Here's how the part is built. I have some questions about the finished solid (model axes, mm). A direction names the side the tool comes from. Round coordinates to 2 decimals unless told otherwise and drop trailing zeros. Write each loop counter-clockwise with the first axis right and the second up, starting at its lowest first coordinate (ties: lowest second). Pieces come first, ordered by that corner, then holes. Notation, with made-up numbers: (68, 78) -> (105, 78) arc R16 ccw to (105, 102) -> close; hole circle Ø3 at (-16.5, -23). An arc over 180 degrees is marked (long way). Answer as CSV lines item,"result".
from build123d import *

# Parameters (mm, degrees)
SKETCH_1_R          = 13.5
SKETCH_1_R_2        = 1.6
EXTRUDE_1_DEPTH     = 3
CUT_EXTRUDE_START   = -10
CUT_EXTRUDE_1_DEPTH = 10
SKETCH_3_W          = 59.8
SKETCH_3_H          = 5
EXTRUDE_1_2_DEPTH   = 3
FILLET_1_R          = 2
SKETCH_4_R          = 1.6
CUT_EXTRUDE_2_DEPTH = 10


with BuildPart() as part:
    # 草图1 → Extrude 1 (new body)
    with BuildSketch(Plane(origin=(0, 0, 0), x_dir=(1, 0, 0), z_dir=(0, 1, 0))):
        with BuildLine():
            Line((-49, -44), (49, -44))
            ThreePointArc((49, -44), (70, -65), (49, -86))
            Line((49, -86), (-49, -86))
            ThreePointArc((-49, -86), (-70, -65), (-49, -44))
        make_face()
        with Locations(Location((-49, -65, 0), (0, 0, 270))):
            Circle(SKETCH_1_R, mode=Mode.SUBTRACT)
        with Locations(Location((49, -65, 0), (0, 0, 270))):
            Circle(SKETCH_1_R, mode=Mode.SUBTRACT)
        with Locations(Location((-49, -82.5, 0), (0, 0, 270))):
            Circle(SKETCH_1_R_2, mode=Mode.SUBTRACT)
        with Locations(Location((-57.75, -80.155444566, 0), (0, 0, 270))):
            Circle(SKETCH_1_R_2, mode=Mode.SUBTRACT)
        with Locations(Location((-64.155444566, -73.75, 0), (0, 0, 270))):
            Circle(SKETCH_1_R_2, mode=Mode.SUBTRACT)
        with Locations(Location((-66.5, -65, 0), (0, 0, 270))):
            Circle(SKETCH_1_R_2, mode=Mode.SUBTRACT)
        with Locations(Location((-64.155444566, -56.25, 0), (0, 0, 270))):
            Circle(SKETCH_1_R_2, mode=Mode.SUBTRACT)
        with Locations(Location((-57.75, -49.844555434, 0), (0, 0, 270))):
            Circle(SKETCH_1_R_2, mode=Mode.SUBTRACT)
        with Locations(Location((-49, -47.5, 0), (0, 0, 270))):
            Circle(SKETCH_1_R_2, mode=Mode.SUBTRACT)
        with Locations(Location((-40.25, -49.844555434, 0), (0, 0, 270))):
            Circle(SKETCH_1_R_2, mode=Mode.SUBTRACT)
        with Locations(Location((-33.844555434, -56.25, 0), (0, 0, 270))):
            Circle(SKETCH_1_R_2, mode=Mode.SUBTRACT)
        with Locations(Location((-31.5, -65, 0), (0, 0, 270))):
            Circle(SKETCH_1_R_2, mode=Mode.SUBTRACT)
        with Locations(Location((-33.844555434, -73.75, 0), (0, 0, 270))):
            Circle(SKETCH_1_R_2, mode=Mode.SUBTRACT)
        with Locations(Location((-40.25, -80.155444566, 0), (0, 0, 270))):
            Circle(SKETCH_1_R_2, mode=Mode.SUBTRACT)
        with Locations(Location((64.155444566, -56.25, 0), (0, 0, 270))):
            Circle(SKETCH_1_R_2, mode=Mode.SUBTRACT)
        with Locations(Location((66.5, -65, 0), (0, 0, 270))):
            Circle(SKETCH_1_R_2, mode=Mode.SUBTRACT)
        with Locations(Location((64.155444566, -73.75, 0), (0, 0, 270))):
            Circle(SKETCH_1_R_2, mode=Mode.SUBTRACT)
        with Locations(Location((57.75, -80.155444566, 0), (0, 0, 270))):
            Circle(SKETCH_1_R_2, mode=Mode.SUBTRACT)
        with Locations(Location((49, -82.5, 0), (0, 0, 270))):
            Circle(SKETCH_1_R_2, mode=Mode.SUBTRACT)
        with Locations(Location((40.25, -80.155444566, 0), (0, 0, 270))):
            Circle(SKETCH_1_R_2, mode=Mode.SUBTRACT)
        with Locations(Location((33.844555434, -73.75, 0), (0, 0, 270))):
            Circle(SKETCH_1_R_2, mode=Mode.SUBTRACT)
        with Locations(Location((31.5, -65, 0), (0, 0, 270))):
            Circle(SKETCH_1_R_2, mode=Mode.SUBTRACT)
        with Locations(Location((33.844555434, -56.25, 0), (0, 0, 270))):
            Circle(SKETCH_1_R_2, mode=Mode.SUBTRACT)
        with Locations(Location((40.25, -49.844555434, 0), (0, 0, 270))):
            Circle(SKETCH_1_R_2, mode=Mode.SUBTRACT)
        with Locations(Location((49, -47.5, 0), (0, 0, 270))):
            Circle(SKETCH_1_R_2, mode=Mode.SUBTRACT)
        with Locations(Location((57.75, -49.844555434, 0), (0, 0, 270))):
            Circle(SKETCH_1_R_2, mode=Mode.SUBTRACT)
        with Locations(Location((13, -52, 0), (0, 0, 270))):
            Circle(SKETCH_1_R_2, mode=Mode.SUBTRACT)
        with Locations(Location((-13, -52, 0), (0, 0, 270))):
            Circle(SKETCH_1_R_2, mode=Mode.SUBTRACT)
        with Locations(Location((13, -78, 0), (0, 0, 270))):
            Circle(SKETCH_1_R_2, mode=Mode.SUBTRACT)
        with Locations(Location((-13, -78, 0), (0, 0, 270))):
            Circle(SKETCH_1_R_2, mode=Mode.SUBTRACT)
    extrude(amount=EXTRUDE_1_DEPTH)

    # 草图2 → 切除-拉伸1 (cut)
    with BuildSketch(Plane(origin=(0, 3, 0), x_dir=(1, 0, 0), z_dir=(0, 1, 0)).offset(CUT_EXTRUDE_START)):
        with BuildLine():
            Line((-16.872983346, -51), (-33.347524158, -51))
            ThreePointArc((-33.347524158, -51), (-29.382380462, -57.506736115), (-28, -65))
            ThreePointArc((-28, -65), (-29.382380462, -72.493263885), (-33.347524158, -79))
            Line((-33.347524158, -79), (-16.872983346, -79))
            ThreePointArc((-16.872983346, -79), (-13.50401717, -74.031881215), (-9, -78))
            ThreePointArc((-9, -78), (-9.031881215, -78.50401717), (-9.127016654, -79))
            Line((-9.127016654, -79), (9.127016654, -79))
            ThreePointArc((9.127016654, -79), (12.49598283, -74.031881215), (17, -78))
            ThreePointArc((17, -78), (16.968118785, -78.50401717), (16.872983346, -79))
            Line((16.872983346, -79), (33.347524158, -79))
            ThreePointArc((33.347524158, -79), (28, -65), (33.347524158, -51))
            Line((33.347524158, -51), (16.872983346, -51))
            ThreePointArc((16.872983346, -51), (16.968118785, -51.49598283), (17, -52))
            ThreePointArc((17, -52), (12.49598283, -55.968118785), (9.127016654, -51))
            Line((9.127016654, -51), (-9.127016654, -51))
            ThreePointArc((-9.127016654, -51), (-9.031881215, -51.49598283), (-9, -52))
            ThreePointArc((-9, -52), (-13.50401717, -55.968118785), (-16.872983346, -51))
        make_face()
        with BuildLine():
            ThreePointArc((17, -78), (12.49598283, -74.031881215), (9.127016654, -79))
            Line((9.127016654, -79), (11.7510004, -79))
            ThreePointArc((11.7510004, -79), (12.470094046, -76.490298149), (14.6, -78))
            ThreePointArc((14.6, -78), (14.509701851, -78.529905954), (14.2489996, -79))
            Line((14.2489996, -79), (16.872983346, -79))
            ThreePointArc((16.872983346, -79), (16.968118785, -78.50401717), (17, -78))
        make_face()
        with BuildLine():
            Line((11.7510004, -79), (9.127016654, -79))
            ThreePointArc((9.127016654, -79), (13, -82), (16.872983346, -79))
            Line((16.872983346, -79), (14.2489996, -79))
            ThreePointArc((14.2489996, -79), (13, -79.6), (11.7510004, -79))
        make_face()
        with BuildLine():
            ThreePointArc((-9.127016654, -51), (-13, -48), (-16.872983346, -51))
            Line((-16.872983346, -51), (-14.2489996, -51))
            ThreePointArc((-14.2489996, -51), (-13, -50.4), (-11.7510004, -51))
            Line((-11.7510004, -51), (-9.127016654, -51))
        make_face()
        with BuildLine():
            Line((-14.2489996, -51), (-16.872983346, -51))
            ThreePointArc((-16.872983346, -51), (-13.50401717, -55.968118785), (-9, -52))
            ThreePointArc((-9, -52), (-9.031881215, -51.49598283), (-9.127016654, -51))
            Line((-9.127016654, -51), (-11.7510004, -51))
            ThreePointArc((-11.7510004, -51), (-11.490298149, -51.470094046), (-11.4, -52))
            ThreePointArc((-11.4, -52), (-13.529905954, -53.509701851), (-14.2489996, -51))
        make_face()
        with BuildLine():
            ThreePointArc((16.872983346, -51), (13, -48), (9.127016654, -51))
            Line((9.127016654, -51), (11.7510004, -51))
            ThreePointArc((11.7510004, -51), (13, -50.4), (14.2489996, -51))
            Line((14.2489996, -51), (16.872983346, -51))
        make_face()
        with BuildLine():
            Line((11.7510004, -51), (9.127016654, -51))
            ThreePointArc((9.127016654, -51), (12.49598283, -55.968118785), (17, -52))
            ThreePointArc((17, -52), (16.968118785, -51.49598283), (16.872983346, -51))
            Line((16.872983346, -51), (14.2489996, -51))
            ThreePointArc((14.2489996, -51), (14.509701851, -51.470094046), (14.6, -52))
            ThreePointArc((14.6, -52), (12.470094046, -53.509701851), (11.7510004, -51))
        make_face()
        with BuildLine():
            ThreePointArc((-9, -78), (-13.50401717, -74.031881215), (-16.872983346, -79))
            Line((-16.872983346, -79), (-14.2489996, -79))
            ThreePointArc((-14.2489996, -79), (-13.529905954, -76.490298149), (-11.4, -78))
            ThreePointArc((-11.4, -78), (-11.490298149, -78.529905954), (-11.7510004, -79))
            Line((-11.7510004, -79), (-9.127016654, -79))
            ThreePointArc((-9.127016654, -79), (-9.031881215, -78.50401717), (-9, -78))
        make_face()
        with BuildLine():
            Line((-14.2489996, -79), (-16.872983346, -79))
            ThreePointArc((-16.872983346, -79), (-13, -82), (-9.127016654, -79))
            Line((-9.127016654, -79), (-11.7510004, -79))
            ThreePointArc((-11.7510004, -79), (-13, -79.6), (-14.2489996, -79))
        make_face()
    extrude(amount=CUT_EXTRUDE_1_DEPTH, mode=Mode.SUBTRACT)

    # 草图3 → Extrude 1 2 (add)
    with BuildSketch(Plane(origin=(0, 3, 0), x_dir=(1, 0, 0), z_dir=(0, 1, 0))):
        with Locations((0, -65)):
            Rectangle(SKETCH_3_W, SKETCH_3_H)
    extrude(amount=-EXTRUDE_1_2_DEPTH)

    # 圆角1
    fillet_1_edges = [part.edges().sort_by_distance(p)[0] for p in [
        (-33.347524158, 1.5, 79),
        (-33.347524158, 1.5, 51),
        (-16.872983346, 1.5, 51),
        (-9.127016654, 1.5, 51),
        (9.127016654, 1.5, 51),
        (16.872983346, 1.5, 51),
        (33.347524158, 1.5, 51),
        (33.347524158, 1.5, 79),
        (16.872983346, 1.5, 79),
        (9.127016654, 1.5, 79),
        (-16.872983346, 1.5, 79),
        (-9.127016654, 1.5, 79),
        (28.149340538, 1.5, 62.5),
        (28.149340538, 1.5, 67.5),
        (-28.149340538, 1.5, 62.5),
        (-28.149340538, 1.5, 67.5),
    ]]
    fillet(fillet_1_edges, radius=FILLET_1_R)

    # 草图4 → 切除-拉伸2 (cut)
    with BuildSketch(Plane(origin=(0, 3, 0), x_dir=(1, 0, 0), z_dir=(0, 1, 0)).offset(CUT_EXTRUDE_START)):
        with Locations(Location((-49, -82.5, 0), (0, 0, 270))):
            Circle(SKETCH_4_R)
        with Locations(Location((-49, -47.5, 0), (0, 0, 270))):
            Circle(SKETCH_4_R)
        with Locations(Location((25, -82.5, 0), (0, 0, 270))):
            Circle(SKETCH_4_R)
        with Locations(Location((-25, -82.5, 0), (0, 0, 270))):
            Circle(SKETCH_4_R)
        with Locations(Location((-25, -47.5, 0), (0, 0, 270))):
            Circle(SKETCH_4_R)
        with Locations(Location((25, -47.5, 0), (0, 0, 270))):
            Circle(SKETCH_4_R)
    extrude(amount=CUT_EXTRUDE_2_DEPTH, mode=Mode.SUBTRACT)


solid = part.part
Item 1: Suppose I cut it at A-A, the plane z = 65. List the corners of the cut face in (x, y) for me, then the cut area to 3 significant figures.
Results found:
outline,"(-70, 0) -> (-68.1, 0) -> (-68.1, 3) -> (-70, 3) -> close; (-64.9, 0) -> (-62.5, 0) -> (-62.5, 3) -> (-64.9, 3) -> close; (-35.5, 0) -> (-33.1, 0) -> (-33.1, 3) -> (-35.5, 3) -> close; (-29.9, 0) -> (29.9, 0) -> (29.9, 3) -> (-29.9, 3) -> close; (33.1, 0) -> (35.5, 0) -> (35.5, 3) -> (33.1, 3) -> close; (62.5, 0) -> (64.9, 0) -> (64.9, 3) -> (62.5, 3) -> close; (68.1, 0) -> (70, 0) -> (70, 3) -> (68.1, 3) -> close"
area,"220 mm²"
Item 2: Will these pins go through, and if not, where does the flat tip stop? pin 1 (3 mm diameter, centred on x = -32.5, z = 78.5, fed in from -Y); pin 2 (2.5 mm diameter, centred on x = 40.25, z = 49.84, fed in from +Y).
Results found:
pin 1,"stops at y = 0"
pin 2,"passes through"
Item 3: I need wall thicknesses on L1, parallel to Z at x = -22, y = 1.75; L2, parallel to X at y = 1.95, z = 82.5; L3, parallel to X at y = 2.4, z = 67. Which ranges of each line are inside material? Lowest first, please.
Results found:
L1,"z = 44 to 51, 62.5 to 67.5, 79 to 86"
L2,"x = -60.61 to -50.6, -47.4 to -26.6, -23.4 to 23.4, 26.6 to 47.4, 50.6 to 60.61"
L3,"x = -69.9 to -62.35, -35.65 to 35.65, 62.35 to 69.9"
Item 4: If we mould it in two halves opening along X, with no side actions, what happens to faces 1 (the cylindrical face through (-29.462, 1.479, 57.301)), 2 (the cylindrical face through (-70, 1, 65)), 3 (the flat face through (1, 0, 65))? For each: pulls with the +X half, pulls with the -X half, needs draft (parallel to the pull), parting line crosses it, or undercut.
Results found:
face 1,"undercut"
face 2,"pulls with the -X half"
face 3,"needs draft"
Item 5: Suppose I cut it at D-D, the plane z = 73.75. State how many separate pieces and enclosed holes the cut face has, then the cut area to 3 significant figures.
Results found:
separate pieces,"8"
enclosed holes,"0"
area,"67.3 mm²"
Item 6: Suppose I cut it at C-C, the plane x = -25. List the corners of the cut face in (y, z) for me, then the cut area to 3 significant figures.
Results found:
outline,"(0, 44) -> (3, 44) -> (3, 45.9) -> (0, 45.9) -> close; (0, 49.1) -> (3, 49.1) -> (3, 51) -> (0, 51) -> close; (0, 62.5) -> (3, 62.5) -> (3, 67.5) -> (0, 67.5) -> close; (0, 79) -> (3, 79) -> (3, 80.9) -> (0, 80.9) -> close; (0, 84.1) -> (3, 84.1) -> (3, 86) -> (0, 86) -> close"
area,"37.8 mm²"
Item 7: For faces 4 (the flat face through (-1, 1, 44)), 5 (the flat face through (0, 1, 79)), which set-ups out of +Z, -Z, +X, -X, +Y, -Y let a thin tool reach every point of the face, with its end or its side?
Results found:
face 4,"-Z, +X, -X, +Y, -Y"
face 5,"+Y, -Y"
Item 8: Suppose I cut it at B-B, the plane x = 0. List the corners of the cut face in (y, z) for me, then the cut area to 3 significant figures.
Results found:
outline,"(0, 44) -> (3, 44) -> (3, 51) -> (0, 51) -> close; (0, 62.5) -> (3, 62.5) -> (3, 67.5) -> (0, 67.5) -> close; (0, 79) -> (3, 79) -> (3, 86) -> (0, 86) -> close"
area,"57.0 mm²"
